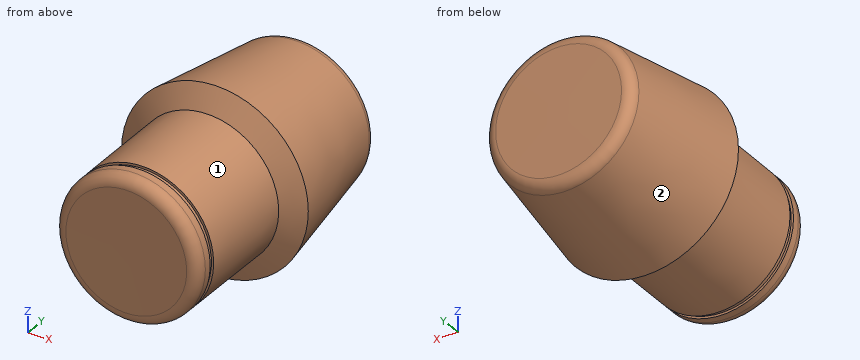
```python
from build123d import *


with BuildPart() as part:
    # Sketch2 → Revolve1 (revolve)
    with BuildSketch(Plane.XY, mode=Mode.PRIVATE) as revolve1_sk:
        with BuildLine():
            Line((0, 0), (6.7564, 0))
            ThreePointArc((6.7564, 0), (7.654425612, 0.371974388), (8.0264, 1.27))
            Line((8.0264, 1.27), (8.0264, 2.102867264))
            Line((8.0264, 2.102867264), (7.7724, 2.102867264))
            Line((7.7724, 2.102867264), (7.7724, 2.709800424))
            Line((7.7724, 2.709800424), (8.0264, 2.709800424))
            Line((8.0264, 2.709800424), (8.0264, 13.97))
            Line((8.0264, 13.97), (10.387716219, 15.438949013))
            Line((10.387716219, 15.438949013), (8.194857048, 29.406966649))
            ThreePointArc((8.194857048, 29.406966649), (7.765679113, 30.175154818), (6.940223979, 30.48))
            Line((6.940223979, 30.48), (-0.1016, 30.48))
            Line((-0.1016, 30.48), (0, 0))
        make_face()
    revolve(revolve1_sk.sketch.rotate(Axis((-0.1016, 30.48, 0), (0.0033333148149691442, -0.9999944444907404, 0)), 180), axis=Axis((-0.1016, 30.48, 0), (0.0033333148149691442, -0.9999944444907404, 0)))


solid = part.part
```
Geometry: final body of the model. Coordinates: model frame, mm. Face numbers are marked on the shaded views. A direction names the side the tool comes from. Give positions to 0.01 mm unless a question says otherwise; leave off trailing zeros. Use CSV: the item, a comma, the result in double quotes.
(1) Ray query, line 1 along Y through (x, z) = (3.75, -2.75); line 2 along Y through (x, z) = (-4, -6.5); line 3 along Z through (x, y) = (-0.25, 28). Return the intervals inside material, ascending. Write a range as [from, to].
From the geometry:
line 1,"[0, 30.48]"
line 2,"[0.31, 30.32]"
line 3,"[-8.5, 8.5]"
(2) First-contact query: P1, Ø10, axis at x = -4.5, z = 4, coming from the +Y side; P2, Ø12, axis at x = 1.5, z = 0.5, coming from the -Y side; P3, Ø8, axis at y = 12, z = -7.5, coming from the -X side. Flat tips, straight axial feed; report the tip coordinate or a pass-through.
From the geometry:
P1,"y = 30.48"
P2,"y = -0.03"
P3,"x = -9.01"
(3) Access query for the marked faces 1 and 2. Directions: +Z, -Z, +X, -X, +Y, -Y. A direction counts if a zero-diameter tool reaches every point of the face in a straight line with its end or side. Return the directions, or none.
From the geometry:
face 1,"-Y"
face 2,"+Y"
